Geometry check sheet. Reference: the model listing, model coordinates, mm. A direction names the side the tool comes from. Give positions to 0.01 mm unless a question says otherwise; leave off trailing zeros. Write each loop counter-clockwise with the first axis right and the second up, starting at its lowest first coordinate (ties: lowest second). Pieces come first, ordered by that corner, then holes.
(1) Mould release check, pull along Y, two halves, no side actions. Record for faces 1 (the cylindrical face through (0.262, 10.23, 1.479)), 2 (the cylindrical face through (-8.73, -0.6, 1.48)), 3 (the cylindrical face through (-8.43, -5.8, 1.48)): +Y half, -Y half, draft (parallel to the pull), parting line (faces both ways), or undercut.
(2) Cross-section at C-C (y = -15). Record the boundary of the cut face in (x, z).
(3) Thickness scan on line 1 along Y through (x, z) = (-9, 1.5); line 2 along Y through (x, z) = (-5.5, 0.95); line 3 along X through (y, z) = (-9.5, 0.4). Record the ranges inside material, lowest first.
(4) Cross-section at B-B (z = 0.85). Count the separate pieces of the cut face and the enclosed holes in it, and give its area (3 significant figures).
(5) Tool access check on faces 4 (the cylindrical face through (-5.619, 6.708, 1.479)), 5 (the cylindrical face through (-1.52, -10.1, 1.48)), 6 (the cylindrical face through (-8.122, 6.225, 1.479)), 7 (the cylindrical face through (-1.674, 10.073, 1.479)). Record the directions out of +Z, -Z, +X, -X, +Y, -Y that give a thin tool (end or side, any length) a straight path to the whole face; none if there is none.
(6) Cross-section at A-A (x = 8). Record the boundary of the cut face in (y, z).
(7) Depth check by flat-ended pin: P1, Ø4, axis at x = 0, y = 0, coming from the +Z side; P2, Ø1.8, axis at x = 19.11, y = -24.04, coming from the -Z side; P3, Ø0.5, axis at y = 9, z = 2, coming from the -X side. Enter the tip coordinate at first touch or a pass-through.
```python
from build123d import *

# Parameters (mm, degrees)
EXTRUSION_DENTS_DEPTH        = 3
R_P_TITION_CIRCULAIRE2_COUNT = 20
ESQUISSE1_R                  = 8.75
EXTRUSION_DISQUE_DEPTH       = 3
BOSS_EXTRU_1_DEPTH           = 3
ESQUISSE6_R                  = 1.5
BOSS_EXTRU_2_DEPTH           = 3
ESQUISSE3_R                  = 1.5
ENL_V_MAT_EXTRU_1_DEPTH      = 35.358346143


with BuildPart() as part:
    # Esquisse2 → Extrusion dents (new body)
    with BuildSketch(Plane.XY):
        with BuildLine():
            Line((0, 9.396926208), (0, 8.75))
            ThreePointArc((0, 8.75), (0.761630034, 8.716789529), (1.517478561, 8.617410215))
            Line((1.517478561, 8.617410215), (1.629672464, 9.254533474))
            ThreePointArc((1.629672464, 9.254533474), (1.517874028, 10.109272502), (1.250299377, 10.928712251))
            ThreePointArc((1.250299377, 10.928712251), (0.956235935, 10.958358127), (0.661482168, 10.980092957))
            ThreePointArc((0.661482168, 10.980092957), (0.25763458, 10.219055101), (0, 9.396926208))
        make_face()
    extrude(amount=EXTRUSION_DENTS_DEPTH)


with BuildPart() as r_p_tition_circulaire2_1:
    # R_p_tition circulaire2: pattern copy
    add(part.part.rotate(Axis((0, 0, 0), (0, 0, 1)), 1 * 360 / R_P_TITION_CIRCULAIRE2_COUNT))


with BuildPart() as r_p_tition_circulaire2_2:
    # R_p_tition circulaire2: pattern copy
    add(part.part.rotate(Axis((0, 0, 0), (0, 0, 1)), 2 * 360 / R_P_TITION_CIRCULAIRE2_COUNT))


with BuildPart() as r_p_tition_circulaire2_3:
    # R_p_tition circulaire2: pattern copy
    add(part.part.rotate(Axis((0, 0, 0), (0, 0, 1)), 3 * 360 / R_P_TITION_CIRCULAIRE2_COUNT))


with BuildPart() as r_p_tition_circulaire2_4:
    # R_p_tition circulaire2: pattern copy
    add(part.part.rotate(Axis((0, 0, 0), (0, 0, 1)), 4 * 360 / R_P_TITION_CIRCULAIRE2_COUNT))


with BuildPart() as r_p_tition_circulaire2_5:
    # R_p_tition circulaire2: pattern copy
    add(part.part.rotate(Axis((0, 0, 0), (0, 0, 1)), 5 * 360 / R_P_TITION_CIRCULAIRE2_COUNT))


with BuildPart() as r_p_tition_circulaire2_6:
    # R_p_tition circulaire2: pattern copy
    add(part.part.rotate(Axis((0, 0, 0), (0, 0, 1)), 6 * 360 / R_P_TITION_CIRCULAIRE2_COUNT))


with BuildPart() as r_p_tition_circulaire2_7:
    # R_p_tition circulaire2: pattern copy
    add(part.part.rotate(Axis((0, 0, 0), (0, 0, 1)), 7 * 360 / R_P_TITION_CIRCULAIRE2_COUNT))


with BuildPart() as r_p_tition_circulaire2_8:
    # R_p_tition circulaire2: pattern copy
    add(part.part.rotate(Axis((0, 0, 0), (0, 0, 1)), 8 * 360 / R_P_TITION_CIRCULAIRE2_COUNT))


with BuildPart() as r_p_tition_circulaire2_9:
    # R_p_tition circulaire2: pattern copy
    add(part.part.rotate(Axis((0, 0, 0), (0, 0, 1)), 9 * 360 / R_P_TITION_CIRCULAIRE2_COUNT))


with BuildPart() as r_p_tition_circulaire2_10:
    # R_p_tition circulaire2: pattern copy
    add(part.part.rotate(Axis((0, 0, 0), (0, 0, 1)), 10 * 360 / R_P_TITION_CIRCULAIRE2_COUNT))


with BuildPart() as r_p_tition_circulaire2_11:
    # R_p_tition circulaire2: pattern copy
    add(part.part.rotate(Axis((0, 0, 0), (0, 0, 1)), 11 * 360 / R_P_TITION_CIRCULAIRE2_COUNT))


with BuildPart() as r_p_tition_circulaire2_12:
    # R_p_tition circulaire2: pattern copy
    add(part.part.rotate(Axis((0, 0, 0), (0, 0, 1)), 12 * 360 / R_P_TITION_CIRCULAIRE2_COUNT))


with BuildPart() as r_p_tition_circulaire2_13:
    # R_p_tition circulaire2: pattern copy
    add(part.part.rotate(Axis((0, 0, 0), (0, 0, 1)), 13 * 360 / R_P_TITION_CIRCULAIRE2_COUNT))


with BuildPart() as r_p_tition_circulaire2_14:
    # R_p_tition circulaire2: pattern copy
    add(part.part.rotate(Axis((0, 0, 0), (0, 0, 1)), 14 * 360 / R_P_TITION_CIRCULAIRE2_COUNT))


with BuildPart() as r_p_tition_circulaire2_15:
    # R_p_tition circulaire2: pattern copy
    add(part.part.rotate(Axis((0, 0, 0), (0, 0, 1)), 15 * 360 / R_P_TITION_CIRCULAIRE2_COUNT))


with BuildPart() as r_p_tition_circulaire2_16:
    # R_p_tition circulaire2: pattern copy
    add(part.part.rotate(Axis((0, 0, 0), (0, 0, 1)), 16 * 360 / R_P_TITION_CIRCULAIRE2_COUNT))


with BuildPart() as r_p_tition_circulaire2_17:
    # R_p_tition circulaire2: pattern copy
    add(part.part.rotate(Axis((0, 0, 0), (0, 0, 1)), 17 * 360 / R_P_TITION_CIRCULAIRE2_COUNT))


with BuildPart() as r_p_tition_circulaire2_18:
    # R_p_tition circulaire2: pattern copy
    add(part.part.rotate(Axis((0, 0, 0), (0, 0, 1)), 18 * 360 / R_P_TITION_CIRCULAIRE2_COUNT))


with BuildPart() as r_p_tition_circulaire2_19:
    # R_p_tition circulaire2: pattern copy
    add(part.part.rotate(Axis((0, 0, 0), (0, 0, 1)), 19 * 360 / R_P_TITION_CIRCULAIRE2_COUNT))


with BuildPart() as part_1:
    add(part.part)

    add(r_p_tition_circulaire2_1.part)  # Extrusion disque merges R_p_tition circulaire2_1

    add(r_p_tition_circulaire2_2.part)  # Extrusion disque merges R_p_tition circulaire2_2

    add(r_p_tition_circulaire2_3.part)  # Extrusion disque merges R_p_tition circulaire2_3

    add(r_p_tition_circulaire2_4.part)  # Extrusion disque merges R_p_tition circulaire2_4

    add(r_p_tition_circulaire2_5.part)  # Extrusion disque merges R_p_tition circulaire2_5

    add(r_p_tition_circulaire2_6.part)  # Extrusion disque merges R_p_tition circulaire2_6

    add(r_p_tition_circulaire2_7.part)  # Extrusion disque merges R_p_tition circulaire2_7

    add(r_p_tition_circulaire2_8.part)  # Extrusion disque merges R_p_tition circulaire2_8

    add(r_p_tition_circulaire2_9.part)  # Extrusion disque merges R_p_tition circulaire2_9

    add(r_p_tition_circulaire2_10.part)  # Extrusion disque merges R_p_tition circulaire2_10

    add(r_p_tition_circulaire2_11.part)  # Extrusion disque merges R_p_tition circulaire2_11

    add(r_p_tition_circulaire2_12.part)  # Extrusion disque merges R_p_tition circulaire2_12

    add(r_p_tition_circulaire2_13.part)  # Extrusion disque merges R_p_tition circulaire2_13

    add(r_p_tition_circulaire2_14.part)  # Extrusion disque merges R_p_tition circulaire2_14

    add(r_p_tition_circulaire2_15.part)  # Extrusion disque merges R_p_tition circulaire2_15

    add(r_p_tition_circulaire2_16.part)  # Extrusion disque merges R_p_tition circulaire2_16

    add(r_p_tition_circulaire2_17.part)  # Extrusion disque merges R_p_tition circulaire2_17

    add(r_p_tition_circulaire2_18.part)  # Extrusion disque merges R_p_tition circulaire2_18

    add(r_p_tition_circulaire2_19.part)  # Extrusion disque merges R_p_tition circulaire2_19
    # Esquisse1 → Extrusion disque (add)
    with BuildSketch(Plane.XY):
        Circle(ESQUISSE1_R)
    extrude(amount=EXTRUSION_DISQUE_DEPTH)

    # Esquisse5 → Boss.-Extru.1 (add)
    with BuildSketch(Plane(origin=(0, 0, 0), x_dir=(-1, 0, 0), z_dir=(0, 0, -1))):
        with BuildLine():
            Line((-0.957126431, 10.958280385), (0.957449481, -10.958252164))
            ThreePointArc((0.957449481, -10.958252164), (-10.958266276, -0.957287956), (-0.957126431, 10.958280385))
        make_face()
    extrude(amount=-BOSS_EXTRU_1_DEPTH)

    # Esquisse6 → Boss.-Extru.2 (add)
    with BuildSketch(Plane(origin=(0, 0, 0), x_dir=(-1, 0, 0), z_dir=(0, 0, -1))):
        with BuildLine():
            Line((-8.621821658, -6.83111933), (-21.064860521, -22.489049712))
            ThreePointArc((-21.064860521, -22.489049712), (-20.662999081, -26.001670868), (-17.150377925, -25.599809428))
            Line((-17.150377925, -25.599809428), (-4.707339063, -9.941879045))
            ThreePointArc((-4.707339063, -9.941879045), (-6.843671374, -8.61186171), (-8.621821658, -6.83111933))
        make_face()
        with Locations((-19.107619223, -24.04442957)):
            Circle(ESQUISSE6_R, mode=Mode.SUBTRACT)
    extrude(amount=-BOSS_EXTRU_2_DEPTH)

    # Esquisse3 → Enl_v. mat.-Extru.1 (cut, through all)
    with BuildSketch(Plane.XY.offset(3)):
        Circle(ESQUISSE3_R)
    extrude(amount=-ENL_V_MAT_EXTRU_1_DEPTH, mode=Mode.SUBTRACT)


solid = part_1.part
```
Reply:
1. face 1: +Y half
1. face 2: undercut
1. face 3: -Y half
2. outline: (8.73, 0) - (15.11, 0) - (15.11, 3) - (8.73, 3) - close
3. line 1: y = -5.9 to -4.64, -2.91 to -1.27, 0 to 1.58, 2.94 to 4.55
3. line 2: y = -7.57 to 6.81, 7.57 to 9.53
3. line 3: x = -4.59 to -3.29, -1.61 to 10.74
4. separate pieces: 1
4. enclosed holes: 2
4. area: 435 mm2
5. face 4: +Z, -Z
5. face 5: +Z, -Z, -Y
5. face 6: +Z, -Z, -X
5. face 7: +Z, -Z, +Y
6. outline: (-14.09, 0) - (7.55, 0) - (7.55, 3) - (-14.09, 3) - close
7. P1: stops at z = 3
7. P2: passes through
7. P3: stops at x = -5.92
